Geometry check sheet. Reference: the model listing, model coordinates, mm. A direction names the side the tool comes from. Give positions to 0.01 mm unless a question says otherwise; leave off trailing zeros. Order: outer loops, then holes, each group sorted by start corner. A loop starts at its lowest first (then second) coordinate and runs counter-clockwise, first axis right, second up. Notation, with made-up numbers: M 71,10.5 L 113,10.5 A18 cw 113,16.5 Z; hole C 53.5,58.5 d3. An arc over 180 degrees is marked long. Put each result on its own line as item: value. Start each with the question number.
Q1. Section check C-C on y = 5. Record the cut outline in (x, z).
Q2. Go/stop test with flat-tipped pins: pin 1 (3 mm diameter, centred on x = 1, z = 67, fed in from +Y); pin 2 (5 mm diameter, centred on x = -2, z = 66.5, fed in from -Y); pin 3 (2 mm diameter, centred on x = 2, z = 16, fed in from -Y); pin 4 (11 mm diameter, centred on x = 0, y = 0, fed in from -Z). Record where each tip stops, or that it passes through.
Q3. Mould release check, pull along Z, two halves, no side actions. Record for faces 1 (the flat face through (0, 8.5, 65)), 2 (the cylindrical face through (3.32, 0.74, -79.03)), 3 (the flat face through (-4, 0, -90)): +Z half, -Z half, draft (parallel to the pull), parting line (faces both ways), or undercut.
Q4. Section check A-A on z = 48. Record the cut outline in (x, y).
Q5. Material ranges on L1, parallel to Y at x = 0, z = -84; L2, parallel to Y at x = -0.75, z = -55; L3, parallel to Y at x = 8, z = -48.5, recorded low to high.
Q6. Section check B-B on x = -6.75. Record the cut outline in (y, z).
Q7. Access from +Z, -Z, +X, -X, +Y, -Y to the whole of each face (thin tool, end or side, straight path). Record for faces 4 (the cylindrical face through (3.32, 0.74, 79.03)), 5 (the flat face through (-4, 0, 90)), 6 (the flat face through (0, -8.5, 65)).
```python
from build123d import *

# Parameters (mm, degrees)
SKIZZE1_R                       = 10
BASIS_LINEAR_AUSTRAGEN_DEPTH    = 90
SKIZZE5_W                       = 10.535653752
SKIZZE5_H                       = 1.5
SCHNITT_LINEAR_AUSTRAGEN1_DEPTH = 10


with BuildPart() as part:
    # Skizze1 → Basis-Linear austragen (new, symmetric)
    with BuildSketch(Plane.XY):
        with Locations(Location((0, 0, 0), (0, 0, 180))):
            Circle(SKIZZE1_R)
    extrude(amount=BASIS_LINEAR_AUSTRAGEN_DEPTH, both=True)

    # Skizze2 → M8 Gewindebohrung1 (revolve, cut)
    with BuildSketch(Plane(origin=(0, 0, 90), x_dir=(0, -1, 0), z_dir=(1, 0, 0))):
        Polygon((0, 0), (0, 24.292926105), (3.4, 22.25), (3.4, 0), align=None)
    m8_gewindebohrung1 = revolve(axis=Axis((0, 0, 96.35), (0, 0, -1)), mode=Mode.SUBTRACT)

    # Skizze5 → Schnitt-Linear austragen1 (cut)
    with BuildSketch(Plane.XY.offset(70)):
        with Locations((0, 9.25)):
            Rectangle(SKIZZE5_W, SKIZZE5_H)
        with Locations((0, -9.25)):
            Rectangle(SKIZZE5_W, SKIZZE5_H)
    extrude(amount=-SCHNITT_LINEAR_AUSTRAGEN1_DEPTH, mode=Mode.SUBTRACT)

    # Spiegeln1: M8 Gewindebohrung1 across plane
    add(m8_gewindebohrung1.mirror(Plane.XY), mode=Mode.SUBTRACT)


solid = part.part
```
Results found:
1. outline: M -8.66,-90 L 8.66,-90 L 8.66,90 L -8.66,90 Z
2. pin 1: stops at y = 8.5
2. pin 2: stops at y = -8.5
2. pin 3: stops at y = -9.95
2. pin 4: stops at z = -90
3. face 1: undercut
3. face 2: draft
3. face 3: -Z half
4. outline: C 0,0 d20
5. L1: y = -10 to -3.4, 3.4 to 10
5. L2: y = -9.97 to 9.97
5. L3: y = -6 to 6
6. outline: M -7.38,-90 L 7.38,-90 L 7.38,90 L -7.38,90 Z
7. face 4: +Z
7. face 5: +Z, +X, -X, +Y, -Y
7. face 6: +X, -X, -Y
